Could you check a few things on this model? Use its own coordinates, in mm. Face numbers are marked on the shaded views. A direction names the side the tool comes from. Round coordinates to 2 decimals unless told otherwise and drop trailing zeros. Order: outer loops, then holes, each group sorted by start corner. A loop starts at its lowest first (then second) coordinate and runs counter-clockwise, first axis right, second up. Notation, with made-up numbers: (39.25, 76.25) -> (93.25, 76.25) arc R24 cw to (93.25, 93.25) -> close; hole circle Ø2 at (73, 61). An arc over 180 degrees is marked (long way). Put each result on its own line as item: value. Start each with the question number.
from build123d import *

# Parameters (mm, degrees)
BOSS_EXTRUDE1_DEPTH = 50.8
SCALE1_SCALE        = 0.5
SKETCH2_R           = 1.3462
CUT_EXTRUDE1_DEPTH  = 57.620860656
SKETCH3_R           = 2.286
CUT_EXTRUDE2_DEPTH  = 57.620860656
CUT_EXTRUDE3_DEPTH  = 2.286
CUT_EXTRUDE4_DEPTH  = 57.620860656
BOSS_EXTRUDE2_DEPTH = 31.75
SKETCH7_R           = 1.3462
CUT_EXTRUDE5_DEPTH  = 5.08


with BuildPart() as part:
    # Sketch1 → Boss-Extrude1 (new body)
    with BuildSketch(Plane(origin=(-34.925, 0, 0), x_dir=(0, 0, -1), z_dir=(1, 0, 0))):
        with BuildLine():
            Line((38.721808668, -36.878639896), (-2.875579258, 78.983230962))
            Line((-2.875579258, 78.983230962), (-10.16, 68.58))
            Line((-10.16, 68.58), (-10.16, 0))
            ThreePointArc((-10.16, 0), (-9.410554147, -3.829761173), (-7.27278137, -7.094522616))
            Line((-7.27278137, -7.094522616), (28.19983171, -43.458429465))
            ThreePointArc((28.19983171, -43.458429465), (36.112120939, -44.408324587), (38.721808668, -36.878639896))
        make_face()
    extrude(amount=-BOSS_EXTRUDE1_DEPTH)


with BuildPart() as part_1:
    # Scale1: scaled about (-60.325, 10.229435701, -8.69743621)
    add(part.part.scale(SCALE1_SCALE).moved(Location((-30.1625, 5.11471785, -4.348718105))))

    # Sketch2 → Cut-Extrude1 (cut, through all)
    with BuildSketch(Plane(origin=(-47.625, 0, 0), x_dir=(0, 0, -1), z_dir=(1, 0, 0))):
        with Locations((20.721378138, -14.397458564)):
            Circle(SKETCH2_R)
    extrude(amount=-CUT_EXTRUDE1_DEPTH, mode=Mode.SUBTRACT)

    # Sketch3 → Cut-Extrude2 (cut, through all)
    with BuildSketch(Plane(origin=(-47.625, 0, 0), x_dir=(0, 0, -1), z_dir=(1, 0, 0))):
        with Locations((4.348718105, 5.11471785)):
            Circle(SKETCH3_R)
    extrude(amount=-CUT_EXTRUDE2_DEPTH, mode=Mode.SUBTRACT)

    # Sketch4 → Cut-Extrude3 (cut, symmetric)
    with BuildSketch(Plane(origin=(-60.325, 0, 0), x_dir=(0, 0, -1), z_dir=(1, 0, 0))):
        with BuildLine():
            Line((9.58048069, -7.52352017), (18.44863396, -16.614496882))
            ThreePointArc((18.44863396, -16.614496882), (22.404778575, -17.089444443), (23.709622439, -13.324602098))
            Line((23.709622439, -13.324602098), (18.502250725, 1.179573745))
            Line((18.502250725, 1.179573745), (9.58048069, -7.52352017))
        make_face()
    extrude(amount=CUT_EXTRUDE3_DEPTH, both=True, mode=Mode.SUBTRACT)

    # Sketch5 → Cut-Extrude4 (cut, through all)
    with BuildSketch(Plane(origin=(-47.625, 0, 0), x_dir=(0, 0, -1), z_dir=(1, 0, 0))):
        Polygon((1.795924155, 43.013942134), (16.43679686, 2.234484886), (17.930919011, 2.770913119), (2.910928476, 44.606333332), align=None)
    extrude(amount=-CUT_EXTRUDE4_DEPTH, mode=Mode.SUBTRACT)

    # Sketch6 → Boss-Extrude2 (add, symmetric)
    with BuildSketch(Plane(origin=(-60.325, 0, 0), x_dir=(0, 0, -1), z_dir=(1, 0, 0))):
        Polygon((-0.731281895, 22.25971785), (-0.731281895, 39.40471785), (1.795924155, 43.013942134), (9.116360508, 22.62421351), align=None)
    extrude(amount=BOSS_EXTRUDE2_DEPTH, both=True)

    # Sketch7 → Cut-Extrude5 (cut)
    # profile 1 of 3: a face of its own
    with BuildSketch(Plane(origin=(-47.625, 0, 0), x_dir=(0, 0, -1), z_dir=(1, 0, 0))):
        with BuildLine():
            ThreePointArc((23.709622439, -13.324602098), (22.075761864, -11.525826672), (19.648521671, -11.409214263))
            ThreePointArc((19.648521671, -11.409214263), (19.037977702, -11.705472686), (18.504339821, -12.124714386))
            ThreePointArc((18.504339821, -12.124714386), (17.546622489, -14.358068573), (18.44863396, -16.614496882))
            ThreePointArc((18.44863396, -16.614496882), (21.918178505, -17.338256735), (23.896378138, -14.397458564))
            ThreePointArc((23.896378138, -14.397458564), (23.849340786, -13.852963686), (23.709622439, -13.324602098))
        make_face()
        with Locations((20.721378138, -14.397458564)):
            Circle(SKETCH7_R, mode=Mode.SUBTRACT)
    # profile 2 of 3: a face of its own
    with BuildSketch(Plane(origin=(-47.625, 0, 0), x_dir=(0, 0, -1), z_dir=(1, 0, 0))):
        with BuildLine():
            ThreePointArc((18.44863396, -16.614496882), (17.546622489, -14.358068573), (18.504339821, -12.124714386))
            Line((18.504339821, -12.124714386), (16.231595643, -14.341752704))
            Line((16.231595643, -14.341752704), (18.44863396, -16.614496882))
        make_face()
    # profile 3 of 3: a face of its own
    with BuildSketch(Plane(origin=(-47.625, 0, 0), x_dir=(0, 0, -1), z_dir=(1, 0, 0))):
        with BuildLine():
            Line((22.636765972, -10.336357797), (19.648521671, -11.409214263))
            ThreePointArc((19.648521671, -11.409214263), (22.075761864, -11.525826672), (23.709622439, -13.324602098))
            Line((23.709622439, -13.324602098), (22.636765972, -10.336357797))
        make_face()
    cut_extrude5 = extrude(amount=-CUT_EXTRUDE5_DEPTH, mode=Mode.SUBTRACT)

    # Mirror1: Cut-Extrude5 across plane
    add(cut_extrude5.mirror(Plane(origin=(-60.325, 0, 0), x_dir=(0, 0, 1), z_dir=(1, 0, 0))), mode=Mode.SUBTRACT)


solid = part_1.part
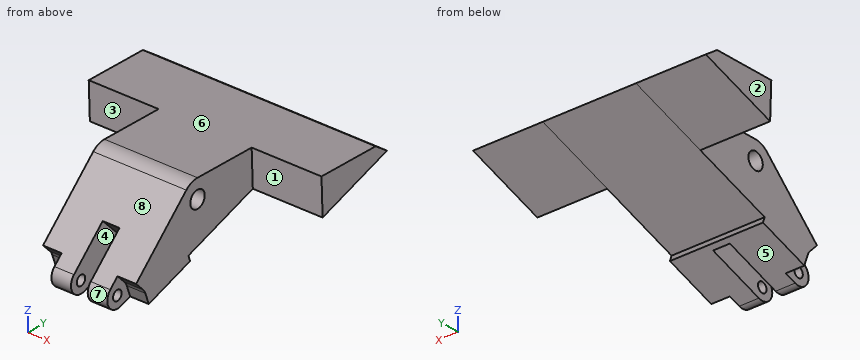
1. If we section it at B-B, the plane x = -51.5: Please give me the cut outline in (y, z) (3 decimals), then the cut area to 3 significant figures.
2. I need wall thicknesses on L1, parallel to X at y = 17, z = -10 (3 decimals); L2, parallel to Z at x = -63, y = 5; L3, parallel to Z at x = -68.5, y = -1.5. Which ranges of each line are inside material? Lowest first, please.
3. If we section it at C-C, the plane y = 4: Please give me the cut outline in (x, z) (3 decimals), then the cut area to 3 significant figures.
4. If we section it at D-D, the plane z = -21.25: Please give me the cut outline in (x, y) (3 decimals), then the cut area to 3 significant figures.
5. Which directions (+Z, -Z, +X, -X, +Y, -Y) give clear straight access to the entire face, cutting with the end or side of a thin tool? Please do the marked faces 1, 2, 3 and 4.
6. If we section it at A-A, the plane z = -5.5: Please give me the cut outline in (x, y) (3 decimals).
7. For pin 1 Ø6 at (y, z) = (5.11, -4.35) entering from +X (3 decimals); pin 2 Ø6 at (x, y) = (-70.5, 9.5) entering from -Z; pin 3 Ø6 at (x, y) = (-58, 27.5) entering from -Z, each with a flat end and sliding along its axis, tell me the tip position at first contact or that it passes through.
8. Thinking about a two-plate mould opening in Y: for the marked faces 5, 6, 7 and 8, which applies, +Y half, -Y half, draft (parallel to the pull), parting line (faces both ways), or undercut?
Results below:
1. outline: (-14.342, -16.232) -> (-12.125, -18.504) arc R3.175 cw to (-11.409, -19.649) -> (-10.336, -22.637) -> (2.771, -17.931) -> (2.234, -16.437) -> (43.014, -1.796) -> (39.405, 0.731) -> (5.115, 0.731) arc R5.08 ccw to (1.567, -0.712) -> close; hole circle Ø4.572 at (5.115, -4.349)
1. area: 576 mm2
2. L1: -73.025 to -47.625
2. L2: -15.44 to -6.63, -2.07 to 0.73
2. L3: -19.46 to -3.7
3. outline: (-73.025, -15.803) -> (-47.625, -15.803) -> (-47.625, -6.345) -> (-73.025, -6.345) -> close; (-73.025, -2.353) -> (-47.625, -2.353) -> (-47.625, 0.607) -> (-73.025, 0.607) -> close
3. area: 315 mm2
4. outline: (-73.025, -10.834) -> (-67.945, -10.834) -> (-67.945, -13.159) -> (-62.611, -13.159) -> (-62.611, -6.474) -> (-73.025, -6.474) -> close; (-67.945, -17.528) -> (-62.611, -17.528) -> (-62.611, -15.636) -> (-67.945, -15.636) -> close; (-58.039, -17.528) -> (-52.705, -17.528) -> (-52.705, -15.636) -> (-58.039, -15.636) -> close; (-58.039, -13.159) -> (-52.705, -13.159) -> (-52.705, -10.834) -> (-47.625, -10.834) -> (-47.625, -6.474) -> (-58.039, -6.474) -> close
4. area: 136 mm2
5. face 1: -Z, +X, -Y
5. face 2: +Z, -Z, -X, +Y, -Y
5. face 3: -Z, -X, -Y
5. face 4: -Z, -Y
6. outline: (-92.075, 22.49) -> (-73.025, 22.49) -> (-73.025, 7.09) -> (-47.625, 7.09) -> (-47.625, 22.49) -> (-28.575, 22.49) -> (-28.575, 32.697) -> (-92.075, 32.697) -> close; (-73.025, -3.341) -> (-47.625, -3.341) -> (-47.625, 3.14) -> (-73.025, 3.14) -> close
7. pin 1: x = -47.625
7. pin 2: z = -14.91
7. pin 3: z = -8.44
8. face 5: +Y half
8. face 6: draft
8. face 7: parting line
8. face 8: -Y half
